Verification items for the finished model (mm, model axes). Give positions to 0.01 mm unless a question says otherwise; leave off trailing zeros. Order: outer loops, then holes, each group sorted by start corner. A loop starts at its lowest first (then second) coordinate and runs counter-clockwise, first axis right, second up. Notation, with made-up numbers: (30.25, -34) - (65.25, -34) arc R8 cw to (65.25, -30) - close; hole circle Ø6 at (-16.5, -30.75). An arc over 180 degrees is marked (long way). Answer as a JSON object with one key per item and string values.
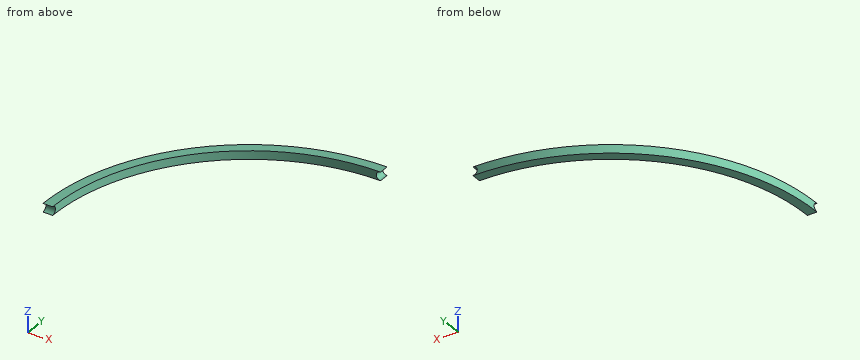
```python
from build123d import *

# Parameters (mm, degrees)
BOSS_EXTRUDE1_DEPTH = 6
SKETCH3_R           = 3
CUT_EXTRUDE1_DEPTH  = 172
SKETCH4_R           = 3
CUT_EXTRUDE2_DEPTH  = 175


with BuildPart() as part:
    # Sketch2 → Boss-Extrude1 (new body)
    with BuildSketch(Plane.XY):
        with BuildLine():
            Line((0, 139.2), (0, 146))
            ThreePointArc((0, 146), (-103.237590053, 103.237590053), (-146, 0))
            Line((-146, 0), (-139.2, 0))
            ThreePointArc((-139.2, 0), (-98.429263941, 98.429263941), (0, 139.2))
        make_face()
    extrude(amount=BOSS_EXTRUDE1_DEPTH)

    # Sketch3 → Cut-Extrude1 (cut)
    with BuildSketch(Plane(origin=(0, 0, 0), x_dir=(0, 0, -1), z_dir=(1, 0, 0))):
        with Locations((-3, 0)):
            Circle(SKETCH3_R)
    extrude(amount=-CUT_EXTRUDE1_DEPTH, mode=Mode.SUBTRACT)

    # Sketch4 → Cut-Extrude2 (cut)
    with BuildSketch(Plane(origin=(0, 0, 0), x_dir=(1, 0, 0), z_dir=(0, 1, 0))):
        with Locations((0, -3)):
            Circle(SKETCH4_R)
    extrude(amount=CUT_EXTRUDE2_DEPTH, mode=Mode.SUBTRACT)


solid = part.part
```
(1) Section check B-B (x = -94). Record the cut outline in (y, z).
Computed values:
{"outline": "(102.67, 0) - (111.71, 0) - (111.71, 6) - (102.67, 6) - close"}
(2) Gauge pin test, flat ends, axial feed: pin 1 Ø3 at (y, z) = (35.5, 2.5) entering from +X; pin 2 Ø2 at (y, z) = (94.5, 1.5) entering from +X; pin 3 Ø8 at (x, y) = (-121, 59.5) entering from -Z; pin 4 Ø1 at (x, z) = (-98.5, 1) entering from -Y. Record the tip position at first contact, or that the pin passes through.
Computed values:
{"pin 1": "stops at x = -134.19", "pin 2": "stops at x = -101.27", "pin 3": "passes through", "pin 4": "stops at y = 97.86"}
(3) Material ranges on line 1 along Y through (x, z) = (-114, 1.5); line 2 along Y through (x, z) = (-90.5, 1); line 3 along X through (y, z) = (62, 0.5), recorded low to high. Write a range as [from, to].
Computed values:
{"line 1": "y = [79.88, 91.21]", "line 2": "y = [105.77, 114.57]", "line 3": "x = [-132.18, -124.63]"}
(4) Section check A-A (y = 48). Record the cut outline in (x, z), then the cut area to 3 significant figures.
Computed values:
{"outline": "(-137.88, 0) - (-130.66, 0) - (-130.66, 6) - (-137.88, 6) - close", "area": "43.3 mm²"}
